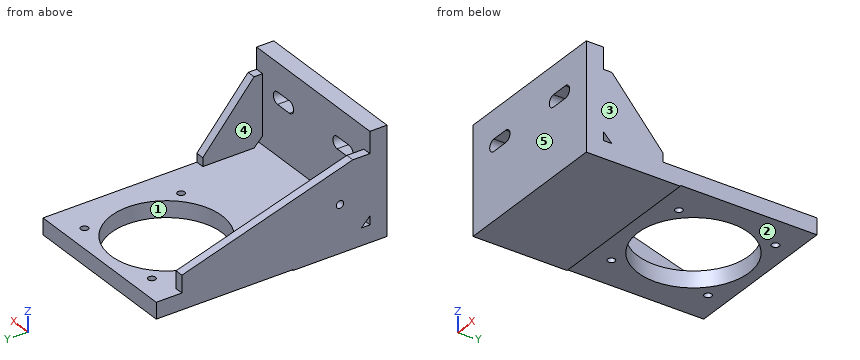
```python
from build123d import *

# Parameters (mm, degrees)
SKETCH1_W                  = 190
SKETCH1_H                  = 125
BOSS_EXTRUDE1_DEPTH        = 20
SKETCH2_W                  = 190
SKETCH2_H                  = 250
BOSS_EXTRUDE2_DEPTH        = 20
SKETCH3_W                  = 80
SKETCH3_H                  = 220
BOSS_EXTRUDE3_DEPTH        = 10
SKETCH4_W                  = 80
SKETCH4_H                  = 70
BOSS_EXTRUDE4_DEPTH        = 10
CUT_EXTRUDE1_DEPTH         = 354.022662162
CUT_EXTRUDE2_DEPTH         = 10
CUT_EXTRUDE3_DEPTH         = 10
SKETCH8_W                  = 190
SKETCH8_H                  = 160
CUT_EXTRUDE4_DEPTH         = 1
SKETCH9_R                  = 65
CUT_EXTRUDE5_DEPTH         = 353.669817251
CUT_EXTRUDE6_DEPTH         = 338.971892322
M10X1_5_TAPPED_HOLE1_D     = 8.5
M10X1_5_TAPPED_HOLE2_D     = 8.5
M10X1_5_TAPPED_HOLE2_DEPTH = 10


with BuildPart() as part:
    # Sketch1 → Boss-Extrude1 (new body)
    with BuildSketch(Plane(origin=(0, 0, 0), x_dir=(1, 0, 0), z_dir=(0, 1, 0))):
        with Locations((95, -62.5)):
            Rectangle(SKETCH1_W, SKETCH1_H)
    extrude(amount=BOSS_EXTRUDE1_DEPTH)

    # Sketch2 → Boss-Extrude2 (add)
    with BuildSketch(Plane(origin=(0, 0, 0), x_dir=(-1, 0, 0), z_dir=(0, 0, -1))):
        with Locations((-95, 145)):
            Rectangle(SKETCH2_W, SKETCH2_H)
    extrude(amount=-BOSS_EXTRUDE2_DEPTH)

    # Sketch3 → Boss-Extrude3 (add)
    with BuildSketch(Plane.ZY):
        with Locations((60, 130)):
            Rectangle(SKETCH3_W, SKETCH3_H)
    extrude(amount=-BOSS_EXTRUDE3_DEPTH)

    # Sketch4 → Boss-Extrude4 (add)
    with BuildSketch(Plane(origin=(190, 0, 0), x_dir=(0, 0, -1), z_dir=(1, 0, 0))):
        with Locations((-60, 55)):
            Rectangle(SKETCH4_W, SKETCH4_H)
    extrude(amount=-BOSS_EXTRUDE4_DEPTH)

    # Sketch5 → Cut-Extrude1 (cut, through all)
    with BuildSketch(Plane.ZY):
        Polygon((20, 30), (20, 20), (30, 20), align=None)
    extrude(amount=-CUT_EXTRUDE1_DEPTH, mode=Mode.SUBTRACT)

    # Sketch6 → Cut-Extrude2 (cut)
    with BuildSketch(Plane.ZY):
        Polygon((40, 240), (100, 40), (100, 240), align=None)
    extrude(amount=-CUT_EXTRUDE2_DEPTH, mode=Mode.SUBTRACT)

    # Sketch7 → Cut-Extrude3 (cut)
    with BuildSketch(Plane(origin=(190, 0, 0), x_dir=(0, 0, -1), z_dir=(1, 0, 0))):
        Polygon((-100, 90), (-30, 90), (-100, 30), align=None)
    extrude(amount=-CUT_EXTRUDE3_DEPTH, mode=Mode.SUBTRACT)

    # Sketch8 → Cut-Extrude4 (cut)
    with BuildSketch(Plane(origin=(0, 0, 0), x_dir=(-1, 0, 0), z_dir=(0, 0, -1))):
        with Locations((-95, 190)):
            Rectangle(SKETCH8_W, SKETCH8_H)
    extrude(amount=-CUT_EXTRUDE4_DEPTH, mode=Mode.SUBTRACT)

    # Sketch9 → Cut-Extrude5 (cut, through all)
    with BuildSketch(Plane(origin=(0, 0, 1), x_dir=(-1, 0, 0), z_dir=(0, 0, -1))):
        with Locations((-95, 191.7)):
            Circle(SKETCH9_R)
    extrude(amount=-CUT_EXTRUDE5_DEPTH, mode=Mode.SUBTRACT)

    # Sketch10 → Cut-Extrude6 (cut, through all)
    with BuildSketch(Plane(origin=(0, 20, 0), x_dir=(1, 0, 0), z_dir=(0, 1, 0))):
        with BuildLine():
            Line((35, -78), (55, -78))
            ThreePointArc((55, -78), (62, -85), (55, -92))
            Line((55, -92), (35, -92))
            ThreePointArc((35, -92), (28, -85), (35, -78))
        make_face()
        with BuildLine():
            Line((135, -78), (155, -78))
            ThreePointArc((155, -78), (162, -85), (155, -92))
            Line((155, -92), (135, -92))
            ThreePointArc((135, -92), (128, -85), (135, -78))
        make_face()
    extrude(amount=-CUT_EXTRUDE6_DEPTH, mode=Mode.SUBTRACT)

    # M10x1.5 Tapped Hole1 (through all)
    with Locations(Plane(origin=(0, 0, 1), x_dir=(-1, 0, 0), z_dir=(0, 0, -1))):
        with Locations((-38.431457505, 248.268542495), (-151.568542495, 248.268542495), (-151.568542495, 135.131457505), (-38.431457505, 135.131457505)):
            Hole(M10X1_5_TAPPED_HOLE1_D / 2)

    # M10x1.5 Tapped Hole2
    with Locations(Plane.ZY):
        with Locations((55, 55)):
            Hole(M10X1_5_TAPPED_HOLE2_D / 2, depth=M10X1_5_TAPPED_HOLE2_DEPTH)


solid = part.part
```
Geometry check sheet. Reference: the model listing, model coordinates, mm. Face numbers are marked on the shaded views. A direction names the side the tool comes from. Round coordinates to 2 decimals unless told otherwise and drop trailing zeros. Order: outer loops, then holes, each group sorted by start corner. A loop starts at its lowest first (then second) coordinate and runs counter-clockwise, first axis right, second up. Notation, with made-up numbers: (3, -39) - (60, -39) arc R20 cw to (60, -10) - close; hole circle Ø7 at (84.25, 12). An arc over 180 degrees is marked (long way). Use a Markdown table: item, result. Add a question column.
1) Section check C-C (y = 46.5). Record the cut outline in (x, z).
2) Thickness scan on line 1 along Z through (x, y) = (150.5, 12.5); line 2 along Y through (x, z) = (13.5, 38.5). Record the ranges inside material, lowest first.
3) Section check D-D (z = 85). Record the cut outline in (x, y), then the cut area to 3 significant figures.
4) Section check B-B (x = 95). Record the cut outline in (y, z), then the cut area to 3 significant figures.
5) Section check A-A (y = 191.7). Record the cut outline in (x, z), then the cut area to 3 significant figures.
6) Set-up check for the marked faces 1 and 2: record each of +Z, -Z, +X, -X, +Y, -Y from which the full face is reachable in a straight line by a thin tool's end or side.
7) Mould release check, pull along X, two halves, no side actions. Record for the marked faces 3, 4 and 5: released by +X, released by -X, zero draft, split by the parting line, or undercut.
8) Gauge pin test, flat ends, axial feed: P1, Ø12, axis at x = 56, y = 132.5, coming from the +Z side; P2, Ø8, axis at x = 183, z = 26, coming from the +Y side; P3, Ø5, axis at x = 3.5, z = 25.5, coming from the +Y side. Record the tip position at first contact, or that the pin passes through.
Established:
| question | item | result |
|---|---|---|
| 1 | outline | (0, 0) - (190, 0) - (190, 80.75) - (180, 80.75) - (180, 20) - (10, 20) - (10, 98.05) - (0, 98.05) - close |
| 2 | line 1 | 0 to 78, 92 to 125 |
| 2 | line 2 | 0 to 20 |
| 3 | outline | (0, 0) - (28, 0) - (28, 20) - (10, 20) - (10, 90) - (0, 90) - close; (62, 0) - (128, 0) - (128, 20) - (62, 20) - close; (162, 0) - (190, 0) - (190, 42.86) - (180, 42.86) - (180, 20) - (162, 20) - close |
| 3 | area | 3,370 mm2 |
| 4 | outline | (0, 0) - (110, 0) - (110, 1) - (126.7, 1) - (126.7, 20) - (20, 20) - (20, 125) - (0, 125) - close; (256.7, 1) - (270, 1) - (270, 20) - (256.7, 20) - close |
| 4 | area | 4,870 mm2 |
| 5 | outline | (0, 1) - (30, 1) - (30, 20) - (10, 20) - (10, 54.49) - (0, 54.49) - close; (160, 1) - (190, 1) - (190, 20) - (160, 20) - close |
| 5 | area | 1,480 mm2 |
| 6 | face 1 | +Z, -Z |
| 6 | face 2 | -Z, +X, -X, +Y |
| 7 | face 3 | released by +X |
| 7 | face 4 | undercut |
| 7 | face 5 | zero draft |
| 8 | P1 | z = 20 |
| 8 | P2 | y = 90 |
| 8 | P3 | y = 240 |
